```python
from build123d import *

# Parameters (mm, degrees)
SKETCH1_W           = 5
SKETCH1_H           = 5
SKETCH1_R           = 1.5
SKETCH1_R_2         = 5
BOSS_EXTRUDE1_DEPTH = 5
FILLET1_R           = 10


with BuildPart() as part:
    # Sketch1 → Boss-Extrude1 (new body)
    with BuildSketch(Plane.XY):
        Polygon((-75, 125), (-90, 125), (-90, -125), (-75, -125), (-75, -130), (-70, -130), (-70, -125), (-66.5, -125), (-66.5, -122), (-67.6, -122), (-67.6, -119.7), (-66.5, -119.7), (-66.5, -115), (-63.5, -115), (-63.5, -119.7), (-62.4, -119.7), (-62.4, -122), (-63.5, -122), (-63.5, -125), (-60, -125), (-60, -130), (-55, -130), (-55, -125), (55, -125), (55, -130), (60, -130), (60, -125), (63.5, -125), (63.5, -122), (62.4, -122), (62.4, -119.7), (63.5, -119.7), (63.5, -115), (66.5, -115), (66.5, -119.7), (67.6, -119.7), (67.6, -122), (66.5, -122), (66.5, -125), (70, -125), (70, -130), (75, -130), (75, -125), (90, -125), (90, 125), (75, 125), (75, 130), (70, 130), (70, 125), (66.5, 125), (66.5, 122), (67.6, 122), (67.6, 119.7), (66.5, 119.7), (66.5, 115), (63.5, 115), (63.5, 119.7), (62.4, 119.7), (62.4, 122), (63.5, 122), (63.5, 125), (60, 125), (60, 130), (55, 130), (55, 95), (-55, 95), (-55, 130), (-60, 130), (-60, 125), (-63.5, 125), (-63.5, 122), (-62.4, 122), (-62.4, 119.7), (-63.5, 119.7), (-63.5, 115), (-66.5, 115), (-66.5, 119.7), (-67.6, 119.7), (-67.6, 122), (-66.5, 122), (-66.5, 125), (-70, 125), (-70, 130), (-75, 130), align=None)
        with Locations((-82.5, -110)):
            Rectangle(SKETCH1_W, SKETCH1_H, mode=Mode.SUBTRACT)
        with Locations((-82.5, -102.5)):
            Circle(SKETCH1_R, mode=Mode.SUBTRACT)
        with Locations((-82.5, -95)):
            Rectangle(SKETCH1_W, SKETCH1_H, mode=Mode.SUBTRACT)
        with Locations((0, -100)):
            Circle(SKETCH1_R_2, mode=Mode.SUBTRACT)
        with Locations((82.5, -110)):
            Rectangle(SKETCH1_W, SKETCH1_H, mode=Mode.SUBTRACT)
        with Locations((82.5, -102.5)):
            Circle(SKETCH1_R, mode=Mode.SUBTRACT)
        with Locations((82.5, -95)):
            Rectangle(SKETCH1_W, SKETCH1_H, mode=Mode.SUBTRACT)
        with BuildLine():
            Line((-65, -18.081635275), (-46.616032283, -18.081635275))
            ThreePointArc((-46.616032283, -18.081635275), (0, -50), (46.616032283, -18.081635275))
            Line((46.616032283, -18.081635275), (65, -18.081635275))
            Line((65, -18.081635275), (65, -95.958016924))
            Line((65, -95.958016924), (24.671083738, -95.958016924))
            ThreePointArc((24.671083738, -95.958016924), (0, -75), (-24.671083738, -95.958016924))
            Line((-24.671083738, -95.958016924), (-65, -95.958016924))
            Line((-65, -95.958016924), (-65, -18.081635275))
        make_face(mode=Mode.SUBTRACT)
        with Locations((-82.5, 95)):
            Rectangle(SKETCH1_W, SKETCH1_H, mode=Mode.SUBTRACT)
        with Locations((-82.5, 102.5)):
            Circle(SKETCH1_R, mode=Mode.SUBTRACT)
        with Locations((-82.5, 110)):
            Rectangle(SKETCH1_W, SKETCH1_H, mode=Mode.SUBTRACT)
        with BuildLine():
            ThreePointArc((23.227291604, -6.040937406), (0, -24), (-23.227291604, -6.040937406))
            Line((-23.227291604, -6.040937406), (-30, 20))
            Line((-30, 20), (-65, 20))
            Line((-65, 20), (-65, 80))
            Line((-65, 80), (65, 80))
            Line((65, 80), (65, 20))
            Line((65, 20), (30, 20))
            Line((30, 20), (23.227291604, -6.040937406))
        make_face(mode=Mode.SUBTRACT)
        with Locations((82.5, 95)):
            Rectangle(SKETCH1_W, SKETCH1_H, mode=Mode.SUBTRACT)
        with Locations((82.5, 102.5)):
            Circle(SKETCH1_R, mode=Mode.SUBTRACT)
        with Locations((82.5, 110)):
            Rectangle(SKETCH1_W, SKETCH1_H, mode=Mode.SUBTRACT)
    extrude(amount=BOSS_EXTRUDE1_DEPTH)

    # Fillet1
    fillet1_edges = [part.edges().sort_by_distance(p)[0] for p in [
        (-65, -18.081635275, 2.5),
        (-65, -95.958016924, 2.5),
        (-24.671083738, -95.958016924, 2.5),
        (24.671083738, -95.958016924, 2.5),
        (65, -95.958016924, 2.5),
        (65, -18.081635275, 2.5),
        (46.616032283, -18.081635275, 2.5),
        (-46.616032283, -18.081635275, 2.5),
        (30, 20, 2.5),
        (65, 20, 2.5),
        (65, 80, 2.5),
        (-65, 80, 2.5),
        (-65, 20, 2.5),
        (-30, 20, 2.5),
        (-55, 95, 2.5),
        (55, 95, 2.5),
        (90, 125, 2.5),
        (90, -125, 2.5),
        (-90, -125, 2.5),
        (-90, 125, 2.5),
    ]]
    fillet(fillet1_edges, radius=FILLET1_R)


solid = part.part
```
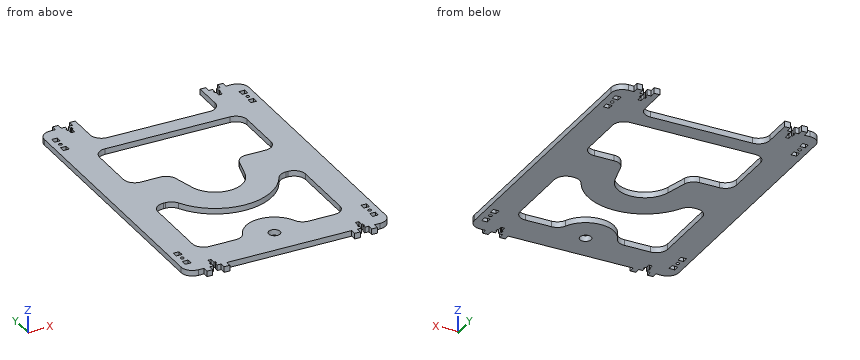
Model file for the job. Use its own axes, mm. Coordinates: 2 decimals unless noted, no trailing zeros. Loops run counter-clockwise (first coordinate to the right, second up) from the corner with the lowest first, then second, coordinate; pieces in that order, holes last. Notation, with made-up numbers: (67, 9.5) - (83, 9.5) arc R23 cw to (83, 44.5) - close; hole circle Ø6 at (25, 77). An arc over 180 degrees is marked (long way). Write item = value, one per line. Start each with the question number.
Item 1: Saw through at B-B, the plane y = -39. List the corners of the cut face in (x, z).
Item 2: Saw through at A-A, the plane x = 0. List the corners of the cut face in (y, z).
Item 3: Drop flat-ended pins along their axis: pin 1 Ø1.5 at (x, z) = (23, 3) entering from -Y; pin 2 Ø1.5 at (x, z) = (-2, 1) entering from +Y; pin 3 Ø1.5 at (y, z) = (-127, 3.5) entering from +X. Give the stop position or say it passes through.
Item 4: Saw through at C-C, the plane z = 2. State how many separate pieces and enclosed holes the cut face has, then the cut area to 3 significant figures.
Item 5: Saw through at D-D, the plane y = -81. List the corners of the cut face in (x, z).
Item 6: Wall check: probe 1 along X at (y, z) = (-110.5, 3.05); probe 2 along X at (y, z) = (-57.5, 3.3); probe 3 along X at (y, z) = (102.5, 2.95). Give the ranges that are in metal, low to high. Write a range as [from, to].
Answers:
q1.outline = (-90, 0) - (-65, 0) - (-65, 5) - (-90, 5) - close; (-31.29, 0) - (31.29, 0) - (31.29, 5) - (-31.29, 5) - close; (65, 0) - (90, 0) - (90, 5) - (65, 5) - close
q2.outline = (-125, 0) - (-105, 0) - (-105, 5) - (-125, 5) - close; (-95, 0) - (-75, 0) - (-75, 5) - (-95, 5) - close; (-50, 0) - (-24, 0) - (-24, 5) - (-50, 5) - close; (80, 0) - (95, 0) - (95, 5) - (80, 5) - close
q3.pin_1 = -125
q3.pin_2 = 95
q3.pin_3 = 75
q4.separate_pieces = 1
q4.enclosed_holes = 15
q4.area = 24,600 mm2
q5.outline = (-90, 0) - (-65, 0) - (-65, 5) - (-90, 5) - close; (-16.25, 0) - (16.25, 0) - (16.25, 5) - (-16.25, 5) - close; (65, 0) - (90, 0) - (90, 5) - (65, 5) - close
q6.probe_1 = [-90, -85], [-80, 80], [85, 90]
q6.probe_2 = [-90, -65], [65, 90]
q6.probe_3 = [-90, -84], [-81, -54.68], [54.68, 81], [84, 90]
